Work out the finished part from the listing and answer in its coordinate system (mm). A direction names the side the tool comes from. Round coordinates to 2 decimals unless told otherwise and drop trailing zeros. Loops run counter-clockwise (first coordinate to the right, second up) from the corner with the lowest first, then second, coordinate; pieces in that order, holes last. Notation, with made-up numbers: (27, 36.5) - (81, 36.5) arc R34 ccw to (81, 71.5) - close; hole circle Ø11 at (81, 2.5). An arc over 180 degrees is marked (long way). Return JSON: item names as keys, results as strings.
from build123d import *

# Parameters (mm, degrees)
SKIZZE1_W                                           = 155.6
SKIZZE1_H                                           = 115.2
AUFSATZ_LINEAR_AUSTRAGEN1_DEPTH                     = 88.8
STIRNSENKUNG_F_R_M8_SENKSCHRAUBE_KOPF_B_D           = 9
STIRNSENKUNG_F_R_M8_SENKSCHRAUBE_KOPF_B_CBORE_D     = 15
STIRNSENKUNG_F_R_M8_SENKSCHRAUBE_KOPF_B_CBORE_DEPTH = 80
SCHNITT_LINEAR_AUSTRAGEN1_DEPTH                     = 189.187566008


with BuildPart() as part:
    # Skizze1 → Aufsatz-Linear austragen1 (new body)
    with BuildSketch(Plane.XY):
        Rectangle(SKIZZE1_W, SKIZZE1_H)
    extrude(amount=AUFSATZ_LINEAR_AUSTRAGEN1_DEPTH)

    # Stirnsenkung für M8 Senkschraube (Kopf Button)1 (through all)
    with Locations(Plane.XY.offset(88.8)):
        with Locations((-47.8, 0)):
            stirnsenkung_f_r_m8_senkschraube_kopf_b = CounterBoreHole(STIRNSENKUNG_F_R_M8_SENKSCHRAUBE_KOPF_B_D / 2, STIRNSENKUNG_F_R_M8_SENKSCHRAUBE_KOPF_B_CBORE_D / 2, STIRNSENKUNG_F_R_M8_SENKSCHRAUBE_KOPF_B_CBORE_DEPTH)

    # Spiegeln1: Stirnsenkung für M8 Senkschraube (Kopf Button)1 across plane
    add(stirnsenkung_f_r_m8_senkschraube_kopf_b.mirror(Plane(origin=(0, 0, 0), x_dir=(0, 0, 1), z_dir=(1, 0, 0))), mode=Mode.SUBTRACT)

    # Skizze6 → Schnitt-Linear austragen1 (cut, through all)
    with BuildSketch(Plane.ZY.offset(77.8)):
        Polygon((44.4, 57.6), (88.8, -19.303055856), (88.8, 57.6), align=None)
    extrude(amount=-SCHNITT_LINEAR_AUSTRAGEN1_DEPTH, mode=Mode.SUBTRACT)


solid = part.part
1) Section B-B (x = -47.8) is taken. Give the vertices of the cut face in (y, z).
Verdict:
{"outline": "(-57.6, 0) - (-4.5, 0) - (-4.5, 8.8) - (-7.5, 8.8) - (-7.5, 81.99) - (-19.3, 88.8) - (-57.6, 88.8) - close; (4.5, 0) - (57.6, 0) - (57.6, 44.4) - (7.5, 73.33) - (7.5, 8.8) - (4.5, 8.8) - close"}
2) Flat-ended cylindrical pins translate along their axes: pin 1 (7 mm diameter, centred on x = 47.8, y = 0, fed in from +Z); pin 2 (16.5 mm diameter, centred on x = -45.5, y = -0.5, fed in from +Z); pin 3 (12 mm diameter, centred on x = 49, y = -0.5, fed in from +Z); pin 4 (8 mm diameter, centred on x = -57, z = 76.5, fed in from +Y). Find the tip coordinate at first contact, or state that the pin passes through.
Verdict:
{"pin 1": "passes through", "pin 2": "stops at z = 82.71", "pin 3": "stops at z = 8.8", "pin 4": "stops at y = 8.93"}
3) A tool of negligible diameter and unlimited length cuts with its end or side. For faces 1 (the flat face through (-1.089, 19.687, 66.289)), 2 (the flat face through (43, 0, 8.8)), from which of +Z, -Z, +X, -X, +Y, -Y can it reach the whole face along a straight path? Write none if from no direction.
Verdict:
{"face 1": "+Z, +X, -X, +Y", "face 2": "+Z"}
4) Section A-A (z = 19.5) is taken. Give the vertices of the cut face in (x, y).
Verdict:
{"outline": "(-77.8, -57.6) - (77.8, -57.6) - (77.8, 57.6) - (-77.8, 57.6) - close; hole circle Ø15 at (-47.8, 0); hole circle Ø15 at (47.8, 0)"}
5) Section C-C (y = 0) is taken. Give the vertices of the cut face in (x, z).
Verdict:
{"outline": "(-77.8, 0) - (-52.3, 0) - (-52.3, 8.8) - (-55.3, 8.8) - (-55.3, 77.66) - (-77.8, 77.66) - close; (-43.3, 0) - (43.3, 0) - (43.3, 8.8) - (40.3, 8.8) - (40.3, 77.66) - (-40.3, 77.66) - (-40.3, 8.8) - (-43.3, 8.8) - close; (52.3, 0) - (77.8, 0) - (77.8, 77.66) - (55.3, 77.66) - (55.3, 8.8) - (52.3, 8.8) - close"}
6) Find the intervals of material crossed by L1, parallel to X at y = 0, z = 30; L2, parallel to Y at x = -47, z = 30; L3, parallel to X at y = -4, z = 32, in increasing order.
Verdict:
{"L1": "x = -77.8 to -55.3, -40.3 to 40.3, 55.3 to 77.8", "L2": "y = -57.6 to -7.46, 7.46 to 57.6", "L3": "x = -77.8 to -54.14, -41.46 to 41.46, 54.14 to 77.8"}
7) Section D-D (x = -10) is taken. Give the vertices of the cut face in (y, z), and give its area (3 significant figures).
Verdict:
{"outline": "(-57.6, 0) - (57.6, 0) - (57.6, 44.4) - (-19.3, 88.8) - (-57.6, 88.8) - close", "area": "8,520 mm2"}
8) Determine the mould class of faces 3 (the cylindrical face through (44.339, -6.654, 45.957)), 4 (the flat face through (-1, -38, 88.8)), 5 (the flat face through (-77.8, -1, 34)) for opening direction X: pulls with the +X half, pulls with the -X half, needs draft (parallel to the pull), parting line crosses it, or undercut.
Verdict:
{"face 3": "undercut", "face 4": "needs draft", "face 5": "pulls with the -X half"}
